CAD build for the part. Positions are in the model's coordinates, mm. A direction names the side the tool comes from. Coordinates: 2 decimals unless noted, no trailing zeros. Loops run counter-clockwise (first coordinate to the right, second up) from the corner with the lowest first, then second, coordinate; pieces in that order, holes last. Notation, with made-up numbers: (48, 36) -> (71, 36) arc R5 cw to (71, 45) -> close; hole circle Ø3 at (75, 21). An arc over 180 degrees is marked (long way). Answer as a JSON object with one key per item and string values. Group by question number.
from build123d import *

# Parameters (mm, degrees)
F0_W      = 67.1
F0_H      = 120
F1_DEPTH  = 3.55
F2_T      = -2.54
F3_R      = 5.08
F4_R      = 5.08
F5_R      = 5.08
F6_R      = 5.08
F7_W      = 22.950821
F7_H      = 8.032788
F8_DEPTH  = 12.5
F9_W      = 25.217273
F9_H      = 3.016623
F10_DEPTH = 12.5


with BuildPart() as f1:
    # F0 (on Front) → F1 (new body, symmetric)
    with BuildSketch(Plane.XZ):
        Rectangle(F0_W, F0_H)
    extrude(amount=F1_DEPTH, both=True)

    # F2
    f2_openings = [f1.faces().sort_by_distance(p)[0] for p in [
        (0, -3.55, 0),
    ]]
    offset(amount=F2_T, openings=f2_openings)

    # F3
    f3_edges = [f1.edges().sort_by_distance(p)[0] for p in [
        (33.55, 0, 60),
    ]]
    fillet(f3_edges, radius=F3_R)

    # F4
    f4_edges = [f1.edges().sort_by_distance(p)[0] for p in [
        (-33.55, 0, 60),
    ]]
    fillet(f4_edges, radius=F4_R)

    # F5
    f5_edges = [f1.edges().sort_by_distance(p)[0] for p in [
        (-33.55, 0, -60),
    ]]
    fillet(f5_edges, radius=F5_R)

    # F6
    f6_edges = [f1.edges().sort_by_distance(p)[0] for p in [
        (33.55, 0, -60),
    ]]
    fillet(f6_edges, radius=F6_R)

    # F7 (on Front) → F8 (cut, symmetric)
    with BuildSketch(Plane.XZ):
        with Locations((18.934428, 61.823776)):
            Rectangle(F7_W, F7_H)
    extrude(amount=F8_DEPTH, both=True, mode=Mode.SUBTRACT)

    # F9 (on face) → F10 (cut, symmetric)
    with BuildSketch(Plane(origin=(0, 0, -60), x_dir=(1, 0, 0), z_dir=(0, 0, -1))):
        with Locations((0.109307, 1.508312)):
            Rectangle(F9_W, F9_H)
    extrude(amount=F10_DEPTH, both=True, mode=Mode.SUBTRACT)


solid = f1.part
Item 1: Drill centre lines: L1, parallel to Z at x = -16.5, y = -2.5; L2, parallel to X at y = 0, z = -13.5; L3, parallel to Z at x = 26.5, y = 0.5. Where is each one in solid material? Low to high.
Item 2: Band-saw the part on A-A, the plane x = -7. List the corners of the cut face in (y, z).
Item 3: Band-saw the part on B-B, the plane z = 16. List the corners of the cut face in (x, y).
Item 4: Band-saw the part on D-D, the plane x = 11. List the corners of the cut face in (y, z), and give its area (3 significant figures).
Item 5: 3-axis set-ups, long thin cutter, end or side, ignore diameter. For faces 5 (the flat face through (0, -1, 57.46)), 6 (the cylindrical face through (32.716, 0.05, 57.709)), 7 (the flat face through (12.718, -1, -59)): which of +Z, -Z, +X, -X, +Y, -Y reach the whole face in a straight line?
Item 6: Band-saw the part on C-C, the plane x = -24. List the corners of the cut face in (y, z), and give its area (3 significant figures).
Item 7: Flat gauge pins, fed straight in: P1, Ø2, axis at y = -2, z = -58, coming from the +X side; P2, Ø4, axis at x = 0, z = -43, coming from the -Y side; P3, Ø1.3, axis at y = -1, z = -58.5, coming from the -X side. Where does each tip first touch, or does it go through?
Item 8: Pull direction Z, two halves, no side cores. Call faces 1 (the flat face through (7.459, 0, 59)), 2 (the flat face through (-0.4, 0.2, -57.46)), 3 (the flat face through (0, 1, -60)), 4 (the flat face through (19, 0, 57.807)): +Z half, -Z half, draft (parallel to the pull), parting line (faces both ways), or undercut.
Reply:
{
 "1": {"L1": "-60 to -57.46, 57.46 to 60", "L2": "-33.55 to -31.01, 31.01 to 33.55", "L3": "-60 to -57.46, 57.46 to 57.81"},
 "2": {"outline": "(-3.55, -60) -> (-3.02, -60) -> (-3.02, -57.46) -> (-3.55, -57.46) -> close; (-3.55, 57.46) -> (1.01, 57.46) -> (1.01, -57.46) -> (0, -57.46) -> (0, -60) -> (3.55, -60) -> (3.55, 60) -> (-3.55, 60) -> close"},
 "3": {"outline": "(-33.55, -3.55) -> (-31.01, -3.55) -> (-31.01, 1.01) -> (31.01, 1.01) -> (31.01, -3.55) -> (33.55, -3.55) -> (33.55, 3.55) -> (-33.55, 3.55) -> close"},
 "4": {"outline": "(-3.55, -60) -> (-3.02, -60) -> (-3.02, -57.46) -> (-3.55, -57.46) -> close; (-3.55, 57.46) -> (1.01, 57.46) -> (1.01, -57.46) -> (0, -57.46) -> (0, -60) -> (3.55, -60) -> (3.55, 57.81) -> (-3.55, 57.81) -> close", "area": "305 mm²"},
 "5": {"face 5": "-Y", "face 6": "+Z, +X, +Y, -Y", "face 7": "-Z"},
 "6": {"outline": "(-3.55, -60) -> (3.55, -60) -> (3.55, 60) -> (-3.55, 60) -> (-3.55, 57.46) -> (1.01, 57.46) -> (1.01, -57.46) -> (-3.55, -57.46) -> close", "area": "328 mm²"},
 "7": {"P1": "x = 33.1", "P2": "y = 1.01", "P3": "x = -32.62"},
 "8": {"face 1": "draft", "face 2": "undercut", "face 3": "-Z half", "face 4": "+Z half"}
}
